Geometry check sheet. Reference: the model listing, model coordinates, mm. A direction names the side the tool comes from. Give positions to 0.01 mm unless a question says otherwise; leave off trailing zeros. Write each loop counter-clockwise with the first axis right and the second up, starting at its lowest first coordinate (ties: lowest second). Pieces come first, ordered by that corner, then holes.
(1) Mould release check, pull along Y, two halves, no side actions. Record for faces 1 (the cylindrical face through (-2.175, -9.794, 5.643)), 2 (the flat face through (-11, 1, 0)), 3 (the flat face through (-22, 3.175, 6)), 4 (the conical face through (13, -1, 11)): +Y half, -Y half, draft (parallel to the pull), parting line (faces both ways), or undercut.
(2) Depth check by flat-ended pin: P1, Ø5, axis at x = 5.5, y = 9, coming from the +Z side; P2, Ø1.5, axis at y = -4.5, z = 9, coming from the -X side; P3, Ø2, axis at x = 5.5, z = 5.5, coming from the +Y side; P4, Ø5, axis at y = 6.5, z = 1.5, coming from the -X side. Enter the tip coordinate at first touch or a pass-through.
(3) Cross-section at C-C (x = -23). Record the boundary of the cut face in (y, z) (3 decimals).
(4) Cross-section at B-B (y = 0). Record the boundary of the cut face in (x, z), and give its area (3 significant figures).
(5) Cross-section at D-D (z = 1.5). Record the boundary of the cut face in (x, y) (3 decimals), and give its area (3 significant figures).
(6) Cross-section at A-A (x = 0). Record the boundary of the cut face in (y, z).
(7) Thickness scan on line 1 along Y through (x, z) = (0, 8.5); line 2 along Y through (x, z) = (-28.5, 6.25) (3 decimals); line 3 along X through (y, z) = (9, 6.75). Record the ranges inside material, lowest first.
(8) Tool access check on faces 5 (the cylindrical face through (13.2, -0.5, 5.6)), 6 (the flat face through (-22, -3.175, 6)). Record the directions out of +Z, -Z, +X, -X, +Y, -Y that give a thin tool (end or side, any length) a straight path to the whole face; none if there is none.
```python
from build123d import *

# Parameters (mm, degrees)
F0_R     = 10.033
F1_DEPTH = 11.43
F2_SIZE  = 0.6


with BuildPart() as f1:
    # F0 (on Top) → F1 (new body)
    with BuildSketch(Plane.XY):
        with BuildLine():
            Line((-31.75, -3.175), (-12.820711, -3.175))
            ThreePointArc((-12.820711, -3.175), (13.208, 0), (-12.820711, 3.175))
            Line((-12.820711, 3.175), (-31.75, 3.175))
            Line((-31.75, 3.175), (-31.75, -3.175))
        make_face()
        Circle(F0_R, mode=Mode.SUBTRACT)
    extrude(amount=F1_DEPTH)

    # F2
    f2_edges = [f1.edges().sort_by_distance(p)[0] for p in [
        (-10.033, 0, 11.43),
        (13.208, 0, 11.43),
        (-22.285356, -3.175, 11.43),
        (-22.285356, 3.175, 11.43),
        (-22.285356, -3.175, 0),
        (-31.75, -3.175, 5.715),
        (13.208, 0, 0),
        (-10.033, 0, 0),
        (-22.285356, 3.175, 0),
        (-31.75, 0, 0),
    ]]
    chamfer(f2_edges, length=F2_SIZE)


solid = f1.part
```
Reply:
1. face 1: undercut
1. face 2: draft
1. face 3: +Y half
1. face 4: parting line
2. P1: stops at z = 11.43
2. P2: stops at x = -12.66
2. P3: stops at y = 12.42
2. P4: stops at x = -12.59
3. outline: (-3.175, 0.6) - (-2.575, 0) - (2.575, 0) - (3.175, 0.6) - (3.175, 10.83) - (2.575, 11.43) - (-2.575, 11.43) - (-3.175, 10.83) - close
4. outline: (-31.75, 0.6) - (-31.15, 0) - (-10.63, 0) - (-10.03, 0.6) - (-10.03, 10.83) - (-10.63, 11.43) - (-31.75, 11.43) - close; (10.03, 0.6) - (10.63, 0) - (12.61, 0) - (13.21, 0.6) - (13.21, 10.83) - (12.61, 11.43) - (10.63, 11.43) - (10.03, 10.83) - close
4. area: 283 mm2
5. outline: (-31.75, -2.575) - (-31.15, -3.175) - (-12.821, -3.175) arc R13.208 ccw (long way) to (-12.821, 3.175) - (-31.75, 3.175) - close; hole circle Ø20.066 at (0, 0)
5. area: 350 mm2
6. outline: (-13.21, 0.6) - (-12.61, 0) - (-10.63, 0) - (-10.03, 0.6) - (-10.03, 10.83) - (-10.63, 11.43) - (-12.61, 11.43) - (-13.21, 10.83) - close; (10.03, 0.6) - (10.63, 0) - (12.61, 0) - (13.21, 0.6) - (13.21, 10.83) - (12.61, 11.43) - (10.63, 11.43) - (10.03, 10.83) - close
7. line 1: y = -13.21 to -10.03, 10.03 to 13.21
7. line 2: y = -3.175 to 3.175
7. line 3: x = -9.67 to -4.43, 4.43 to 9.67
8. face 5: +Z, -Z
8. face 6: +Z, -Z, -X, -Y
